CAD build for the part. Positions are in the model's coordinates, mm. Face numbers are marked on the shaded views. A direction names the side the tool comes from. Coordinates: 2 decimals unless noted, no trailing zeros. Order: outer loops, then holes, each group sorted by start corner. A loop starts at its lowest first (then second) coordinate and runs counter-clockwise, first axis right, second up.
from build123d import *

# Parameters (mm, degrees)
SKETCH1_R               = 19
PISTON_DEPTH            = 5
SKETCH2_R               = 7.9375
ROD_DEPTH               = 36.028
ROD_END_CHAMFER_SIZE    = 1
WRENCH_FLATS_DEPTH      = 45.944596828
WRENCH_FLATS_DEPTH_BACK = 45.944596828


with BuildPart() as part:
    # Sketch1 → Piston (new body)
    with BuildSketch(Plane.XY):
        Circle(SKETCH1_R)
    extrude(amount=PISTON_DEPTH)

    # Sketch2 → Rod (add)
    with BuildSketch(Plane(origin=(0, 0, 0), x_dir=(-1, 0, 0), z_dir=(0, 0, -1))):
        Circle(SKETCH2_R)
    extrude(amount=-ROD_DEPTH)

    # Rod End Chamfer
    rod_end_chamfer_edges = [part.edges().sort_by_distance(p)[0] for p in [
        (7.9375, 0, 36.028),
    ]]
    chamfer(rod_end_chamfer_edges, length=ROD_END_CHAMFER_SIZE)

    # Sketch11 → Wrench Flats (cut, two sides: drawn at the far end of the back side and taken through both)
    with BuildSketch(Plane(origin=(0, 0, 0), x_dir=(1, 0, 0), z_dir=(0, 1, 0)).offset(-WRENCH_FLATS_DEPTH_BACK)):
        Polygon((-6.35, -36.028), (-6.35, -33.028), (-11.35, -30.141248654), (-11.35, -36.028), align=None)
        Polygon((6.35, -36.028), (6.35, -33.028), (11.35, -30.141248654), (11.35, -36.028), align=None)
    extrude(amount=WRENCH_FLATS_DEPTH + WRENCH_FLATS_DEPTH_BACK, mode=Mode.SUBTRACT)


solid = part.part
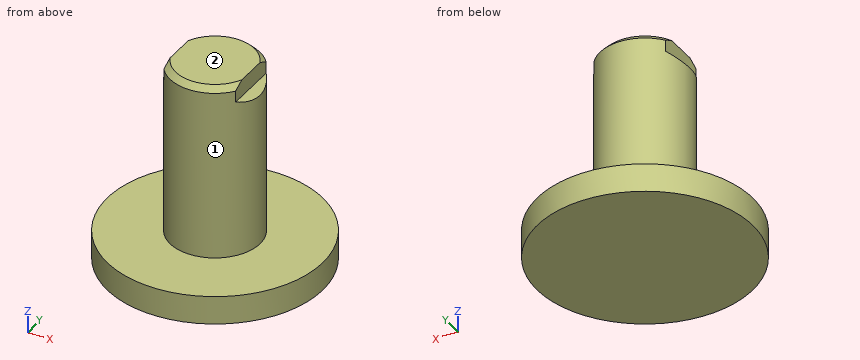
1) Which spindle directions (+Z, -Z, +X, -X, +Y, -Y) get a long thin tool onto all of the face, cutting with end or side? Do the marked faces 1 and 2. Say none if no direction does.
2) Slice it at C-C (z = 14.5). List the corners of the cut face in (x, y) (1 decimal).
3) Slice it at A-A (x = 0). List the corners of the cut face in (y, z), plus the area to 3 significant figures.
4) Slice it at D-D (x = 15). List the corners of the cut face in (y, z), plus the area to 3 significant figures.
5) Slice it at B-B (y = 0). List the corners of the cut face in (x, z), plus the area to 3 significant figures.
6) Drill centre lines: probe 1 along Z at (x, y) = (-10, 14); probe 2 along Y at (x, z) = (-3.5, 32.5); probe 3 along Y at (x, z) = (-4, 19). Where is each one in solid material? Low to high.
7) Pin check, flat tips, straight feed: P1, Ø1, axis at x = 7, z = 26.5, coming from the +Y side; P2, Ø6, axis at y = 8.5, z = 15, coming from the +X side; P3, Ø2.5, axis at y = 0, z = 34, coming from the -X side; P4, Ø6, axis at x = -11.5, z = 31.5, coming from the -Y side. Stop position of each tip, or through.
Worked out:
1. face 1: +Z
1. face 2: +Z, +X, -X, +Y, -Y
2. outline: circle Ø15.9 at (0, 0)
3. outline: (-19, 0) - (19, 0) - (19, 5) - (7.94, 5) - (7.94, 35.03) - (6.94, 36.03) - (-6.94, 36.03) - (-7.94, 35.03) - (-7.94, 5) - (-19, 5) - close
3. area: 682 mm2
4. outline: (-11.66, 0) - (11.66, 0) - (11.66, 5) - (-11.66, 5) - close
4. area: 117 mm2
5. outline: (-19, 0) - (19, 0) - (19, 5) - (7.94, 5) - (7.94, 32.11) - (6.35, 33.03) - (6.35, 36.03) - (-6.35, 36.03) - (-6.35, 33.03) - (-7.94, 32.11) - (-7.94, 5) - (-19, 5) - close
5. area: 672 mm2
6. probe 1: z = 0 to 5
6. probe 2: y = -7.12 to 7.12
6. probe 3: y = -6.86 to 6.86
7. P1: stops at y = 4.56
7. P2: stops at x = 5.72
7. P3: stops at x = -6.83
7. P4: passes through
